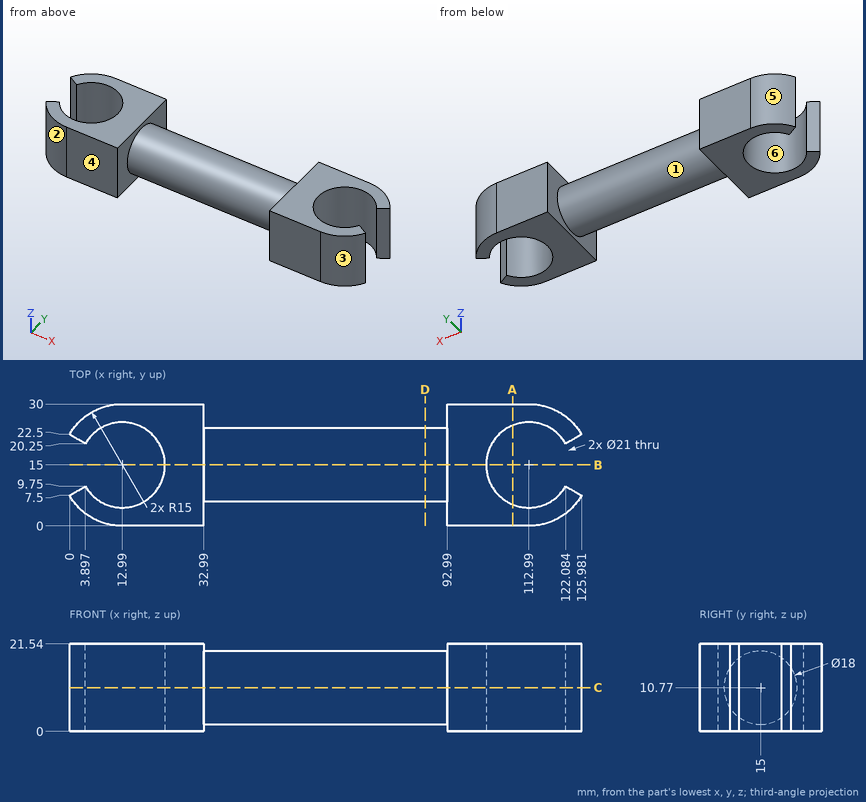
Here's the drawing with two shaded views (mm, measured from the low corner). I have some questions. A direction names the side the tool comes from. Coordinates: 2 decimals unless noted, no trailing zeros. Loops run counter-clockwise (first coordinate to the right, second up) from the corner with the lowest first, then second, coordinate; pieces in that order, holes last. Notation, with made-up numbers: (-21.75, -38) -> (27.25, -38) arc R21 cw to (27.25, -24) -> close; hole circle Ø9 at (75.5, 38). An arc over 180 degrees is marked (long way). Answer in a Markdown table with one row per item.
(1) Imagine slicing it at D-D (x = 87.5). List the corners of the cut face in (y, z) for me.
Results found:
| item | result |
|---|---|
| outline | circle Ø18 at (15, 10.77) |
(2) If I drill on probe 1 along X at (y, z) = (24.25, 13) (1 decimal); probe 2 along X at (y, z) = (23.25, 12.75) (1 decimal); probe 3 along X at (y, z) = (15, 5), over which ranges is the centre line in solid material (lowest first)?
Results found:
| item | result |
|---|---|
| probe 1 | x = 1.2 to 8, 18 to 33, 93 to 108, 118 to 124.8 |
| probe 2 | x = 0.5 to 6.5, 19.5 to 106.5, 119.5 to 125.5 |
| probe 3 | x = 23.49 to 102.49 |
(3) Will these pins go through, and if not, where does the flat tip stop? pin 1 Ø2 at (x, z) = (40, 11.5) entering from -Y; pin 2 Ø8 at (x, y) = (56.5, 18) entering from +Z; pin 3 Ø12 at (x, z) = (89.5, 2.5) entering from +Y; pin 4 Ø10 at (x, z) = (61, 2.5) entering from -Y (1 decimal).
Results found:
| item | result |
|---|---|
| pin 1 | stops at y = 6 |
| pin 2 | stops at z = 19.77 |
| pin 3 | stops at y = 30 |
| pin 4 | stops at y = 6.6 |
(4) Imagine slicing it at C-C (z = 10.77). List the corners of the cut face in (x, y) for me.
Results found:
| item | result |
|---|---|
| outline | (0, 7.5) arc R15 ccw to (12.99, 0) -> (32.99, 0) -> (32.99, 6) -> (92.99, 6) -> (92.99, 0) -> (112.99, 0) arc R15 ccw to (125.98, 7.5) -> (122.08, 9.75) arc R10.5 cw (long way) to (122.08, 20.25) -> (125.98, 22.5) arc R15 ccw to (112.99, 30) -> (92.99, 30) -> (92.99, 24) -> (32.99, 24) -> (32.99, 30) -> (12.99, 30) arc R15 ccw to (0, 22.5) -> (3.9, 20.25) arc R10.5 cw (long way) to (3.9, 9.75) -> close |
(5) Imagine slicing it at A-A (x = 109). List the corners of the cut face in (y, z) for me, plus the area to 3 significant figures.
Results found:
| item | result |
|---|---|
| outline | (0, 0) -> (5.29, 0) -> (5.29, 21.54) -> (0, 21.54) -> close; (24.71, 0) -> (30, 0) -> (30, 21.54) -> (24.71, 21.54) -> close |
| area | 228 mm^2 |
(6) For the marked faces 1 and 2, which set-ups out of +Z, -Z, +X, -X, +Y, -Y let a thin tool reach every point of the face, with its end or its side?
Results found:
| item | result |
|---|---|
| face 1 | none |
| face 2 | +Z, -Z, -X, -Y |
(7) Imagine slicing it at B-B (y = 15). List the corners of the cut face in (x, z) for me, plus the area to 3 significant figures.
Results found:
| item | result |
|---|---|
| outline | (23.49, 0) -> (32.99, 0) -> (32.99, 1.77) -> (92.99, 1.77) -> (92.99, 0) -> (102.49, 0) -> (102.49, 21.54) -> (92.99, 21.54) -> (92.99, 19.77) -> (32.99, 19.77) -> (32.99, 21.54) -> (23.49, 21.54) -> close |
| area | 1,490 mm^2 |
(8) Thinking about a two-plate mould opening in X: for the marked faces 3, 4, 5 and 6, which applies, released by +X, released by -X, zero draft, split by the parting line, or undercut?
Results found:
| item | result |
|---|---|
| face 3 | released by +X |
| face 4 | zero draft |
| face 5 | released by -X |
| face 6 | undercut |
